```python
from build123d import *

# Parameters (mm, degrees)
SKETCH1_W           = 27.7
SKETCH1_H           = 26.77
BOSS_EXTRUDE1_DEPTH = 1.2
SKETCH2_R           = 6.065
BOSS_EXTRUDE2_DEPTH = 10
BOSS_EXTRUDE2_TAPER = 5
SKETCH3_R           = 2.065
CUT_EXTRUDE1_DEPTH  = 9
CHAMFER1_SIZE       = 1.5
CHAMFER1_SIZE_2     = 2.084645451
SKETCH4_R           = 0.875
CUT_EXTRUDE2_DEPTH  = 9


with BuildPart() as part:
    # Sketch1 → Boss-Extrude1 (new body)
    with BuildSketch(Plane(origin=(0, 0, 0), x_dir=(1, 0, 0), z_dir=(0, 1, 0))):
        Rectangle(SKETCH1_W, SKETCH1_H)
    extrude(amount=BOSS_EXTRUDE1_DEPTH)

    # Sketch2 → Boss-Extrude2 (add)
    with BuildSketch(Plane(origin=(0, 1.2, 0), x_dir=(1, 0, 0), z_dir=(0, 1, 0))):
        Circle(SKETCH2_R)
    extrude(amount=BOSS_EXTRUDE2_DEPTH, taper=BOSS_EXTRUDE2_TAPER)

    # Sketch3 → Cut-Extrude1 (cut)
    with BuildSketch(Plane(origin=(0, 11.2, 0), x_dir=(1, 0, 0), z_dir=(0, 1, 0))):
        with Locations(Location((0, 0, 0), (0, 0, 270))):
            Circle(SKETCH3_R)
    extrude(amount=-CUT_EXTRUDE1_DEPTH, mode=Mode.SUBTRACT)

    # Chamfer1
    # the kernel refuses this chamfer: 2.084645451, 1.5 mm, written as the material it adds along each edge
    with BuildSketch(Plane(origin=(0, 1.2, 0), x_dir=(1, 0, 0), z_dir=(0, 0, 1))) as chamfer1_piece_1:
        Polygon((6.065 + CHAMFER1_SIZE, 0), (6.065 - CHAMFER1_SIZE_2 * 0.0871557427277, CHAMFER1_SIZE_2 * 0.996194697864), (6.065, 0), align=None)
    revolve(axis=Axis((0, 1.2, 0), (0, 1, 0)))
    # the kernel refuses this chamfer: 2.084645451, 1.5 mm, written as the material it takes off along each edge
    with BuildSketch(Plane(origin=(0, 11.2, 0), x_dir=(1, 0, 0), z_dir=(0, 0, -1))) as chamfer1_2_piece_1:
        Polygon((5.190113365 + CHAMFER1_SIZE * 0.0871557427477, CHAMFER1_SIZE * 0.996194698092), (5.190113365 - CHAMFER1_SIZE_2, 0), (5.190113365, 0), align=None)
    revolve(axis=Axis((0, 11.2, 0), (0, -1, 0)), mode=Mode.SUBTRACT)

    # Sketch4 → Cut-Extrude2 (cut)
    with BuildSketch(Plane.XY):
        with Locations(Location((0, 6.2, 0), (0, 0, 90.000000002))):
            Circle(SKETCH4_R)
    extrude(amount=CUT_EXTRUDE2_DEPTH, mode=Mode.SUBTRACT)


solid = part.part
```
The model under review builds one solid part; all positions refer to its coordinate system, in mm. A direction names the side the tool comes from. Round coordinates to 2 decimals unless told otherwise and drop trailing zeros. Loops run counter-clockwise (first coordinate to the right, second up) from the corner with the lowest first, then second, coordinate; pieces in that order, holes last. Notation, with made-up numbers: M 30.25,8.5 L 56.25,8.5 A37 ccw 56.25,46.5 Z; hole C 51.25,66.25 d7. An arc over 180 degrees is marked long. Put each result on its own line as item: value.
Q1. Consider section A-A, the plane x = 0. Give the boundary of the cut face in (y, z) (3 decimals).
Result set:
outline: M 0,-13.385 L 1.2,-13.385 L 1.2,-7.565 L 3.277,-5.883 L 9.706,-5.321 L 11.2,-3.105 L 11.2,-2.065 L 2.2,-2.065 L 2.2,2.065 L 5.325,2.065 L 5.325,5.704 L 3.277,5.883 L 1.2,7.565 L 1.2,13.385 L 0,13.385 Z; M 7.075,2.065 L 11.2,2.065 L 11.2,3.105 L 9.706,5.321 L 7.075,5.551 Z
Q2. Mouldability with a two-part tool opening along X and no side actions: class faces 1 (the flat face through (0, 0, 0)), 2 (the conical face through (-1.2, 7.3, 5.4)), 3 (the cylindrical face through (0.091, 6.763, -2.063)) as released by +X, released by -X, zero draft, split by the parting line, or undercut.
Result set:
face 1: zero draft
face 2: split by the parting line
face 3: undercut
Q3. For pin 1 (1 mm diameter, centred on x = 2, y = 7, fed in from +Z); pin 2 (12 mm diameter, centred on x = -11, z = -9.5, fed in from +Y); pin 3 (1.5 mm diameter, centred on x = -3.5, z = 7, fed in from +Y), all flat-tipped, find the tip position at first contact; note any pin that passes through.
Result set:
pin 1: stops at z = 5.36
pin 2: stops at y = 1.2
pin 3: stops at y = 1.8
Q4. Consider section B-B, the plane z = 8.5. Give the boundary of the cut face in (x, y), then the cut area to 3 significant figures.
Result set:
outline: M -13.85,0 L 13.85,0 L 13.85,1.2 L -13.85,1.2 Z
area: 33.2 mm²
Q5. To check wall thickness, follow L1, parallel to X at y = 9.5, z = -0.5; L2, parallel to Y at x = -8, z = -6.5; L3, parallel to Y at x = 0, z = 3.8 (3 decimals). State the ranges of each line that lie inside material, in increasing order.
Result set:
L1: x = -5.32 to -2, 2 to 5.32
L2: y = 0 to 1.2
L3: y = 0 to 5.325, 7.075 to 10.732
Q6. Machinability: for faces 4 (the flat face through (-6, 1.2, 6)), 5 (the cylindrical face through (0.335, 7.008, 3.76)), 6 (the flat face through (0, 1, -13.385)), which of the approach directions +Z, -Z, +X, -X, +Y, -Y give a long, thin tool a straight path to every point of the face, cutting with its end or side? Answer none if there is none.
Result set:
face 4: +Y
face 5: +Z
face 6: -Z, +X, -X, +Y, -Y
Q7. Consider section C-C, the plane x = 8.75. Give the boundary of the cut face in (y, z) (3 decimals), then the cut area to 3 significant figures.
Result set:
outline: M 0,-13.385 L 1.2,-13.385 L 1.2,13.385 L 0,13.385 Z
area: 32.1 mm²
